```python
from build123d import *

# Parameters (mm, degrees)
F0_W     = 77.725055
F0_H     = 38.264645
F1_DEPTH = 25
F2_R     = 5
F3_W     = 10.249458
F3_H     = 7.003797
F3_W_2   = 11.10358
F3_H_2   = 6.491324
F3_W_3   = 11.957702
F3_H_3   = 14.132324
F4_DEPTH = 5


with BuildPart() as f1:
    # F0 (on Front) → F1 (new body)
    with BuildSketch(Plane.XZ):
        with Locations((-13.49512, -13.496899)):
            Rectangle(F0_W, F0_H)
    extrude(amount=F1_DEPTH)

    # F2
    f2_edges = [f1.edges().sort_by_distance(p)[0] for p in [
        (-52.357648, -25, -13.496899),
        (25.367407, -12.5, 5.635423),
        (-52.357648, -12.5, 5.635423),
        (-13.49512, 0, 5.635423),
        (-13.49512, -25, 5.635423),
        (-13.49512, -25, -32.629222),
        (25.367407, -25, -13.496899),
        (25.367407, -12.5, -32.629222),
        (25.367407, 0, -13.496899),
        (-52.357648, 0, -13.496899),
        (-13.49512, 0, -32.629222),
        (-52.357648, -12.5, -32.629222),
    ]]
    fillet(f2_edges, radius=F2_R)

    # F3 (on face) → F4 (cut)
    with BuildSketch(Plane.XZ.offset(25)):
        with Locations((-36.470987, -4.870271)):
            Rectangle(F3_W, F3_H)
        with Locations((9.566161, -4.614035)):
            Rectangle(F3_W_2, F3_H_2)
        with Locations((-14.434654, -20.56306)):
            Rectangle(F3_W_3, F3_H_3)
    extrude(amount=-F4_DEPTH, mode=Mode.SUBTRACT)


solid = f1.part
```
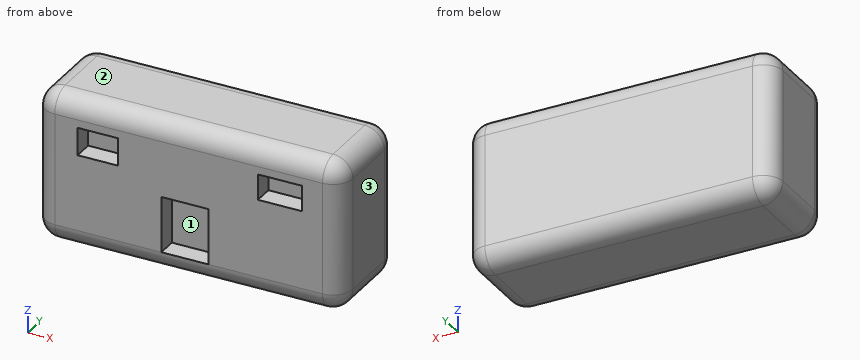
Geometry: final body of the model. Coordinates: model frame, mm. Face numbers are marked on the shaded views. Give positions to 0.01 mm unless a question says otherwise; leave off trailing zeros. Order: outer loops, then holes, each group sorted by start corner. A loop starts at its lowest first (then second) coordinate and runs counter-clockwise, first axis right, second up. Notation, with made-up numbers: M -9.5,37 L 19.5,37 A16 cw 19.5,66 Z; hole C 60.5,23 d5. An arc over 180 degrees is marked long. Answer as CSV lines item,"result". Start each with the question number.
1) Line query: line 1 (X direction, y = -20.75, z = -4.5); line 2 (Y direction, x = -16, z = -20.5); line 3 (X direction, y = -23, z = -19). Output: solid intervals per line, ascending. Write a range as from..to.
2) Cut plane D-D (z = -5.5). Output: boundary loops of the cut face in (x, y), then the cut area to 3 significant figures.
3) Cut plane B-B (y = -21). Output: boundary loops of the cut face in (x, z), then the cut area to 3 significant figures.
4) Cut plane A-A (z = -26). Output: boundary loops of the cut face in (x, y), then the cut area to 3 significant figures.
5) Mould query, pull axis X, two halves, no side actions, for the marked faces 1, 2 and 3. Classes: +X half, -X half, draft (parallel to the pull), parting line (faces both ways), or undercut.
6) First-contact query: P1, Ø1.5, axis at x = -39, y = -22, coming from the +Z side; P2, Ø2.5, axis at x = -14, y = -21.5, coming from the -Z side; P3, Ø5.5, axis at x = -13.5, y = -23, coming from the +Z side; P4, Ø6, axis at y = -4, z = -14.5, coming from the +X side. Flat tips, straight axial feed; report the tip coordinate or a pass-through.
7) Cut plane C-C (x = 7). Output: boundary loops of the cut face in (y, z), then the cut area to 3 significant figures.
Findings below:
1,line 1,"x = -52.3..-41.6, -31.35..4.01, 15.12..25.31"
1,line 2,"y = -20..0"
1,line 3,"x = -51.36..-20.41, -8.46..24.37"
2,outline,"M -52.36,-20 A5 ccw -47.36,-25 L -41.6,-25 L -41.6,-20 L -31.35,-20 L -31.35,-25 L 4.01,-25 L 4.01,-20 L 15.12,-20 L 15.12,-25 L 20.37,-25 A5 ccw 25.37,-20 L 25.37,-5 A5 ccw 20.37,0 L -47.36,0 A5 ccw -52.36,-5 Z"
2,area,"1,810 mm²"
3,outline,"M -52.26,-27.63 A4.9 ccw -47.36,-32.53 L 20.37,-32.53 A4.9 ccw 25.27,-27.63 L 25.27,0.64 A4.9 ccw 20.37,5.53 L -47.36,5.53 A4.9 ccw -52.26,0.64 Z; hole M -41.6,-8.37 L -31.35,-8.37 L -31.35,-1.37 L -41.6,-1.37 Z; hole M -20.41,-27.63 L -8.46,-27.63 L -8.46,-13.5 L -20.41,-13.5 Z; hole M 4.01,-7.86 L 15.12,-7.86 L 15.12,-1.37 L 4.01,-1.37 Z"
3,area,"2,620 mm²"
4,outline,"M -52.36,-20 A5 ccw -47.36,-25 L -20.41,-25 L -20.41,-20 L -8.46,-20 L -8.46,-25 L 20.37,-25 A5 ccw 25.37,-20 L 25.37,-5 A5 ccw 20.37,0 L -47.36,0 A5 ccw -52.36,-5 Z"
4,area,"1,860 mm²"
5,face 1,"undercut"
5,face 2,"draft"
5,face 3,"+X half"
6,P1,"stops at z = 5.48"
6,P2,"stops at z = -32.62"
6,P3,"stops at z = 5.63"
6,P4,"stops at x = 25.37"
7,outline,"M -25,-27.63 A5 ccw -20,-32.63 L -5,-32.63 A5 ccw 0,-27.63 L 0,0.64 A5 ccw -5,5.64 L -20,5.64 A5 ccw -25,0.64 L -25,-1.37 L -20,-1.37 L -20,-7.86 L -25,-7.86 Z"
7,area,"903 mm²"
